```python
from build123d import *

# Parameters (mm, degrees)
SKETCH1_R               = 6.35
BOSS_EXTRUDE1_DEPTH     = 28.575
SKETCH2_W               = 0.924673016
SKETCH2_H               = 0.42538178
BOSS_EXTRUDE3_START     = -43.18
SKETCH7_R               = 6.35
BOSS_EXTRUDE3_DEPTH     = 43.18
SKETCH8_W               = 1.548924628
SKETCH8_H               = 0.472995579
F_1_4_20_TAPPED_HOLE2_D = 5.1054
SKETCH17_W              = 13.324603024
SKETCH17_H              = 8.990077112
CUT_EXTRUDE3_DEPTH      = 0.762


with BuildPart() as part:
    # Sketch1 → Boss-Extrude1 (new body)
    with BuildSketch(Plane(origin=(0, 0, 0), x_dir=(0, 0, -1), z_dir=(1, 0, 0))):
        Circle(SKETCH1_R)
    extrude(amount=BOSS_EXTRUDE1_DEPTH)

    # Sketch2 → Cut-Revolve1 (revolve, cut)
    with BuildSketch(Plane.XY, mode=Mode.PRIVATE) as cut_revolve1_sk:
        with Locations((26.848530558, 6.13730911)):
            Rectangle(SKETCH2_W, SKETCH2_H)
    revolve(cut_revolve1_sk.sketch.rotate(Axis((28.575, 0, 0), (-1, 0, 0)), 90), axis=Axis((28.575, 0, 0), (-1, 0, 0)), mode=Mode.SUBTRACT)

    # Sketch7 → Boss-Extrude3 (add)
    with BuildSketch(Plane(origin=(0, 0, 0), x_dir=(0, 0, -1), z_dir=(1, 0, 0)).offset(BOSS_EXTRUDE3_START)):
        Circle(SKETCH7_R)
    extrude(amount=BOSS_EXTRUDE3_DEPTH)

    # Sketch8 → Cut-Revolve2 (revolve, cut)
    with BuildSketch(Plane.XY, mode=Mode.PRIVATE) as cut_revolve2_sk:
        with Locations((-40.352206887, 6.113502211)):
            Rectangle(SKETCH8_W, SKETCH8_H)
    revolve(cut_revolve2_sk.sketch.rotate(Axis((28.575, 0, 0), (-1, 0, 0)), 90), axis=Axis((28.575, 0, 0), (-1, 0, 0)), mode=Mode.SUBTRACT)

    # 1/4-20 Tapped Hole2 (through all)
    with Locations(Plane(origin=(0, 6.35, 0), x_dir=(1, 0, 0), z_dir=(0, 1, 0))):
        with Locations((-5.36380595, 0)):
            Hole(F_1_4_20_TAPPED_HOLE2_D / 2)

    # Sketch17 → Cut-Extrude3 (cut)
    with BuildSketch(Plane(origin=(0, 6.35, 0), x_dir=(1, 0, 0), z_dir=(0, 1, 0))):
        with Locations((-5.36380595, 0)):
            Rectangle(SKETCH17_W, SKETCH17_H)
    extrude(amount=-CUT_EXTRUDE3_DEPTH, mode=Mode.SUBTRACT)


solid = part.part
```
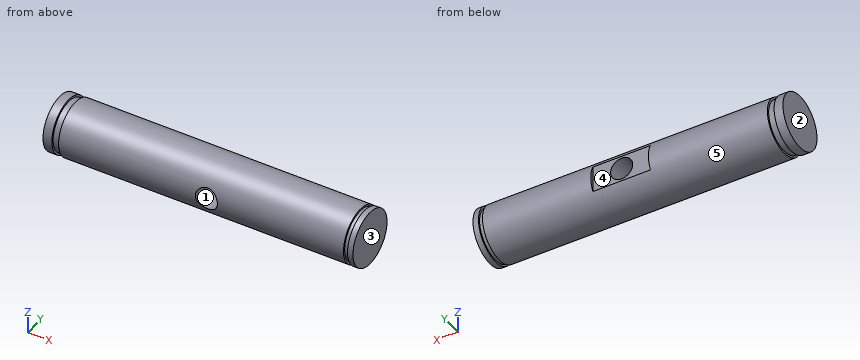
Design review of the part built by this model. Coordinates are the model's own, in mm. Face numbers are marked on the shaded views. A direction names the side the tool comes from. Round coordinates to 2 decimals unless told otherwise and drop trailing zeros. Write each loop counter-clockwise with the first axis right and the second up, starting at its lowest first coordinate (ties: lowest second). Pieces come first, ordered by that corner, then holes.
Item 1: The part is to be moulded in two halves that separate along X. For the marked faces 1, 2 and 3, say which applies: +X half, -X half, draft (parallel to the pull), parting line (faces both ways), or undercut.
Item 2: For the marked faces 4 and 5, list the 3-axis set-ups (+Z, -Z, +X, -X, +Y, -Y) from which the entire face can be reached by the end or side of a thin tool; tool diameter is ignored.
Item 3: Clearance check with flat-ended pins moving along their axes: pin 1 Ø5 at (x, y) = (-5, 4) entering from -Z; pin 2 Ø3 at (x, z) = (4, -5) entering from +Y; pin 3 Ø4 at (x, z) = (16, -4) entering from -Y; pin 4 Ø6 at (x, y) = (-5.5, 0.5) entering from +Z. State where each tip first meets the part, or that it passes through.
Item 4: For probe 1 along X at (y, z) = (3.5, 5.25) (3 decimals); probe 2 along X at (y, z) = (3, 1.5) (3 decimals); probe 3 along X at (y, z) = (-1, 0.5) (3 decimals), list the stretches that pass through material, from the lowest coordinate up.
Item 5: We need section D-D on x = -18. Write out the cut boundary in (y, z).
Item 6: We need section C-C on z = 4. Write out the cut boundary in (x, y) (3 decimals).
Returned:
1. face 1: undercut
1. face 2: -X half
1. face 3: +X half
2. face 4: +Z, -Z, +Y
2. face 5: +X, -X
3. pin 1: stops at z = -6.17
3. pin 2: stops at y = 5.3
3. pin 3: stops at y = -6.03
3. pin 4: stops at z = 6.35
4. probe 1: x = -43.18 to -41.127, -39.578 to 26.386, 27.311 to 28.575
4. probe 2: x = -43.18 to -7.429, -3.298 to 28.575
4. probe 3: x = -43.18 to -7.867, -2.861 to 28.575
5. outline: circle Ø12.7 at (0, 0)
6. outline: (-43.18, -4.932) - (-41.127, -4.932) - (-41.127, -4.306) - (-39.578, -4.306) - (-39.578, -4.932) - (26.386, -4.932) - (26.386, -4.37) - (27.311, -4.37) - (27.311, -4.932) - (28.575, -4.932) - (28.575, 4.932) - (27.311, 4.932) - (27.311, 4.37) - (26.386, 4.37) - (26.386, 4.932) - (-39.578, 4.932) - (-39.578, 4.306) - (-41.127, 4.306) - (-41.127, 4.932) - (-43.18, 4.932) - close
